from build123d import *

# Parameters (mm, degrees)
SKETCH1_W           = 250
SKETCH1_H           = 160
BOSS_EXTRUDE1_DEPTH = 2
CUT_EXTRUDE2_DEPTH  = 50
SKETCH6_W           = 3.552127034
SKETCH6_H           = 144.927795072
CUT_EXTRUDE3_DEPTH  = 50


with BuildPart() as part:
    # Sketch1 → Boss-Extrude1 (new body)
    with BuildSketch(Plane(origin=(0, 0, 0), x_dir=(1, 0, 0), z_dir=(0, 1, 0))):
        Rectangle(SKETCH1_W, SKETCH1_H)
    extrude(amount=BOSS_EXTRUDE1_DEPTH)

    # Sketch5 → Cut-Extrude2 (cut)
    with BuildSketch(Plane(origin=(0, 2, 0), x_dir=(1, 0, 0), z_dir=(0, 1, 0))):
        with BuildLine():
            Line((-125, 40), (-125, 80))
            Line((-125, 80), (-62.5, 80))
            ThreePointArc((-62.5, 80), (-98.97872032, 68.169875501), (-125, 40))
        make_face()
        with BuildLine():
            Line((62.5, 80), (125, 80))
            Line((125, 80), (125, 40))
            ThreePointArc((125, 40), (98.978720329, 68.169875513), (62.5, 80))
        make_face()
        with BuildLine():
            Line((125, -40), (125, -80))
            Line((125, -80), (62.5, -80))
            ThreePointArc((62.5, -80), (98.978720329, -68.169875513), (125, -40))
        make_face()
        with BuildLine():
            Line((-62.5, -80), (-125, -80))
            Line((-125, -80), (-125, -40))
            ThreePointArc((-125, -40), (-99.075756291, -68.321494204), (-62.5, -80))
        make_face()
    extrude(amount=-CUT_EXTRUDE2_DEPTH, mode=Mode.SUBTRACT)

    # Sketch6 → Cut-Extrude3 (cut)
    with BuildSketch(Plane(origin=(0, 2, 0), x_dir=(1, 0, 0), z_dir=(0, 1, 0))):
        with Locations((123.223936483, 4.318146594)):
            Rectangle(SKETCH6_W, SKETCH6_H)
    extrude(amount=-CUT_EXTRUDE3_DEPTH, mode=Mode.SUBTRACT)


solid = part.part
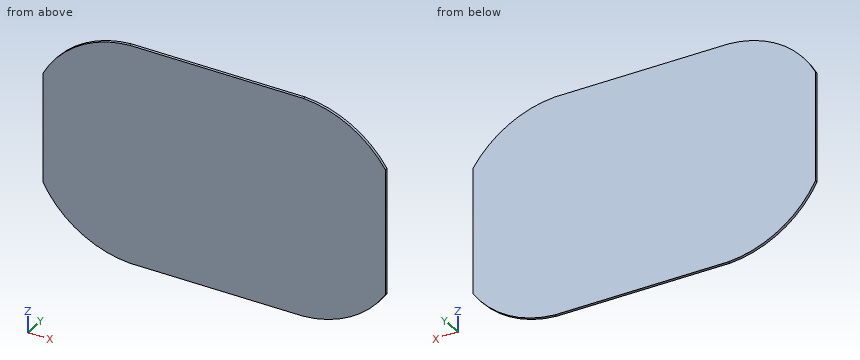
Verification items for the finished model (mm, model axes). Coordinates: 2 decimals unless noted, no trailing zeros. Order: outer loops, then holes, each group sorted by start corner. A loop starts at its lowest first (then second) coordinate and runs counter-clockwise, first axis right, second up. Notation, with made-up numbers: M 15,27.25 L 29,27.25 A7 ccw 29,38.25 Z; hole C 51.5,-32 d8. An arc over 180 degrees is marked long. One line per item, written item: value. Start each with the question number.
Item 1: Gauge pin test, flat end, axial feed: pin 1 (1 mm diameter, centred on x = -64.5, y = 1, fed in from -Z). Record the tip position at first contact, or that the pin passes through.
Item 2: Scan lines: probe 1 along X at (y, z) = (1.2, 50); probe 2 along Z at (x, y) = (101, 1.95); probe 3 along X at (y, z) = (0.7, 58). Record each from-to range of solid material in increasing order.
Item 3: Sectioned sample at B-B (x = 104). Enter the section's corners in (y, z).
Item 4: Sectioned sample at A-A (y = 0.6). Enter the section's corners in (x, z), then the cut area to 3 significant figures.
Item 5: Sectioned sample at C-C (z = 60.5). Enter the section's corners in (x, y).
Conclusion:
1. pin 1: stops at z = -79.9
2. probe 1: x = -118.73 to 118.61
2. probe 2: z = -66.83 to 66.83
2. probe 3: x = -111.85 to 111.64
3. outline: M 0,-64.66 L 2,-64.66 L 2,64.66 L 0,64.66 Z
4. outline: M -125,-40 A75.81 ccw -62.5,-80 L 62.5,-80 A75.81 ccw 121.45,-45.98 L 121.45,45.98 A75.81 ccw 62.5,80 L -62.5,80 A74.61 ccw -125,40 Z
4. area: 36,600 mm^2
5. outline: M -109.25,0 L 109.01,0 L 109.01,2 L -109.25,2 Z
